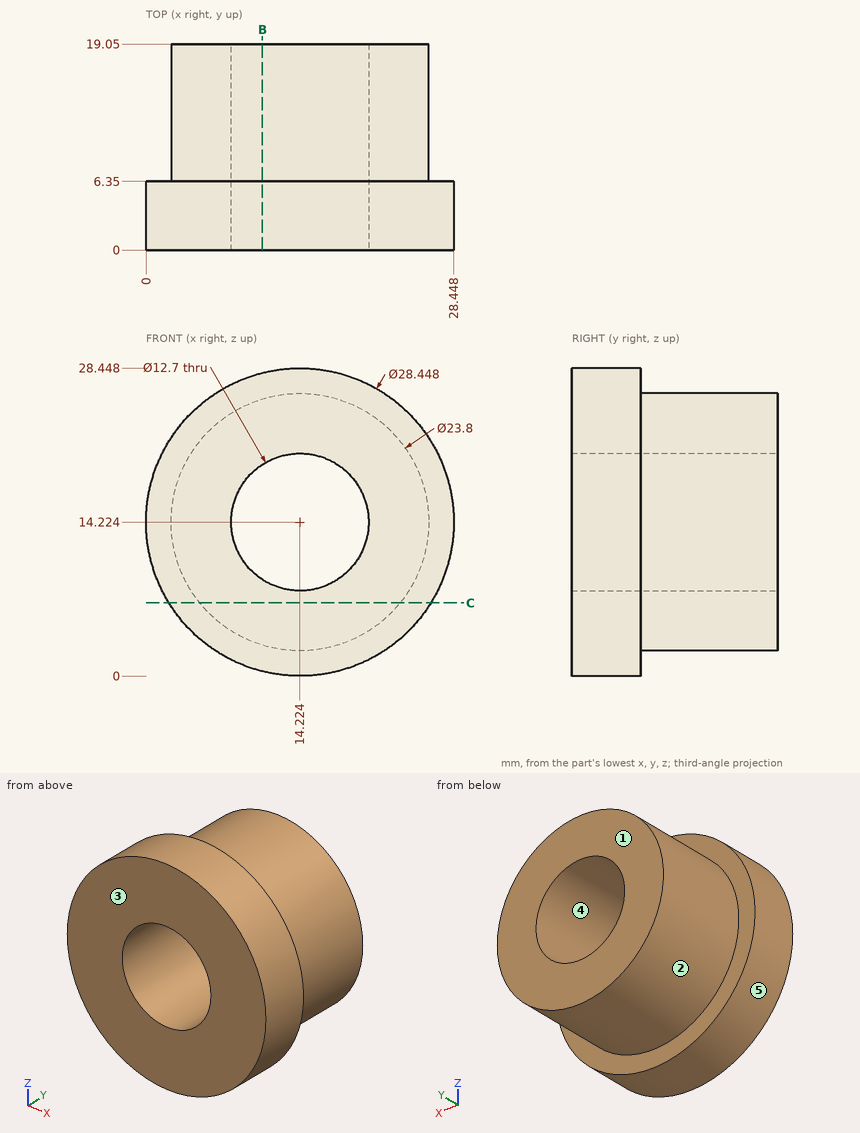
The figure shows three views and two pictorial views of one solid part (mm, origin at its lowest corner). Answer the questions. A direction names the side the tool comes from. Round coordinates to 2 decimals unless told otherwise and drop trailing zeros. Write each loop counter-clockwise with the first axis right and the second up, starting at its lowest first coordinate (ties: lowest second). Pieces come first, ordered by that corner, then holes. Notation, with made-up numbers: M 22.5,59.25 L 55.5,59.25 A29 ccw 55.5,82.25 Z; hole C -19,-37 d9. An arc over 180 degrees is marked long. Write each question's results on one line, items separated by ' | '. Start each with the question number.
(1) Find the intervals of material crossed by line 1 (X direction, y = 7.5, z = 14); line 2 (Y direction, x = 5.25, z = 5.5); line 3 (Z direction, x = 17.75, y = 6) (1 decimal), in increasing order.
(2) The part is cut by section C-C, the plane z = 6.75. Write down the section's boundary in (x, y).
(3) For the marked faces 1 and 2, determine the directions among +Z, -Z, +X, -X, +Y, -Y from which every point of the face is accessible in a straight line to the end or side of a thin tool.
(4) Determine the mould class of the marked faces 3, 4 and 5 for opening direction X: +X half, -X half, draft (parallel to the pull), parting line (faces both ways), or undercut.
(5) Each of these flat-tipped pins is pushed along its axis until it touches: P1, Ø4, axis at y = 8.5, z = 24.5, coming from the +X side (1 decimal); P2, Ø4, axis at x = 22.5, y = 10.5, coming from the +Z side; P3, Ø2, axis at y = 8, z = 23.5, coming from the -X side. Where does it stop, or does it pass through?
(6) The part is cut by section B-B, the plane x = 10.75. Write down the section's boundary in (y, z), and give its area (3 significant figures).
Worked answers:
1) line 1: x = 2.33 to 7.88, 20.57 to 26.12 | line 2: y = 0 to 6.35 | line 3: z = 0.4 to 8.9, 19.5 to 28
2) outline: M 2.12,0 L 26.33,0 L 26.33,6.35 L 23.48,6.35 L 23.48,19.05 L 4.96,19.05 L 4.96,6.35 L 2.12,6.35 Z
3) face 1: +Z, -Z, +X, -X, +Y | face 2: +Y
4) face 3: draft | face 4: undercut | face 5: parting line
5) P1: stops at x = 22.8 | P2: stops at z = 24.33 | P3: stops at x = 5.67
6) outline: M 0,0.43 L 6.35,0.43 L 6.35,2.84 L 19.05,2.84 L 19.05,8.91 L 0,8.91 Z; M 0,19.54 L 19.05,19.54 L 19.05,25.61 L 6.35,25.61 L 6.35,28.02 L 0,28.02 Z | area: 262 mm²
